Part model, mm, in its own coordinate system. Give positions to 0.01 mm unless a question says otherwise; leave off trailing zeros. Write each loop counter-clockwise with the first axis right and the second up, starting at its lowest first coordinate (ties: lowest second). Pieces come first, ordered by that corner, then holes.
```python
from build123d import *

# Parameters (mm, degrees)
SKETCH1_W          = 3
SKETCH1_H          = 64
BASE_FLANGE1_DEPTH = 116
SKETCH3_R          = 2
CUT_EXTRUDE1_DEPTH = 10
FILLET1_R          = 5


# Sheet-metal steps are written as plain solids
with BuildPart() as part:
    # Sketch1 → Base-Flange1 (new body)
    with BuildSketch(Plane.XY):
        with Locations((1.5, 32)):
            Rectangle(SKETCH1_W, SKETCH1_H)
    extrude(amount=BASE_FLANGE1_DEPTH)

    # Sketch3 → Cut-Extrude1 (cut)
    with BuildSketch(Plane.ZY):
        with Locations((18, 60.5)):
            Circle(SKETCH3_R)
        with Locations((98, 60.5)):
            Circle(SKETCH3_R)
        with Locations((98, 3.5)):
            Circle(SKETCH3_R)
        with Locations((18, 3.5)):
            Circle(SKETCH3_R)
    extrude(amount=-CUT_EXTRUDE1_DEPTH, mode=Mode.SUBTRACT)

    # Fillet1
    fillet1_edges = [part.edges().sort_by_distance(p)[0] for p in [
        (1.5, 0, 116),
        (1.5, 0, 0),
        (1.5, 64, 0),
        (1.5, 64, 116),
    ]]
    fillet(fillet1_edges, radius=FILLET1_R)


solid = part.part
```
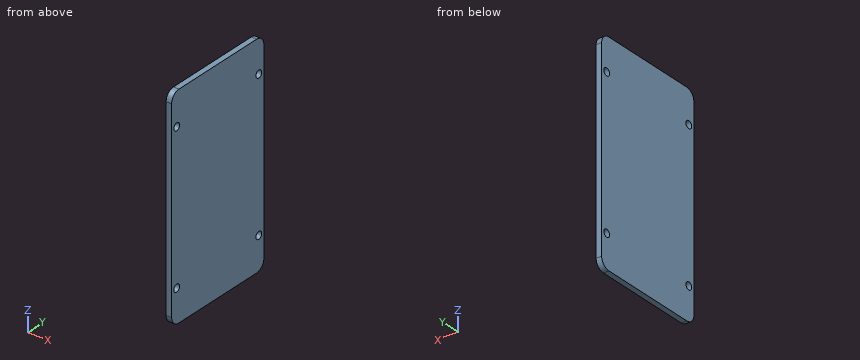
1) Saw through at B-B, the plane y = 3.5. Write the cut outline in (x, z).
Answers follow:
outline: (0, 0.23) - (3, 0.23) - (3, 16) - (0, 16) - close; (0, 20) - (3, 20) - (3, 96) - (0, 96) - close; (0, 100) - (3, 100) - (3, 115.77) - (0, 115.77) - close
2) Wall check: L1, parallel to Y at x = 1.05, z = 98; L2, parallel to Z at x = 0.2, y = 60. Give the ranges that are in metal, low to high.
Answers follow:
L1: y = 0 to 1.5, 5.5 to 58.5, 62.5 to 64
L2: z = 0.1 to 16.06, 19.94 to 96.06, 99.94 to 115.9
3) Saw through at A-A, the plane z = 18. Write the cut outline in (x, y), then the cut area to 3 significant figures.
Answers follow:
outline: (0, 0) - (3, 0) - (3, 1.5) - (0, 1.5) - close; (0, 5.5) - (3, 5.5) - (3, 58.5) - (0, 58.5) - close; (0, 62.5) - (3, 62.5) - (3, 64) - (0, 64) - close
area: 168 mm2
4) Pin check, flat tip, straight feed: pin 1 Ø3 at (y, z) = (3.5, 98) entering from -X. Stop position of the tip, or through.
Answers follow:
pin 1: passes through
